Read the model definition and answer for the solid it produces. Units are mm, in the model's axes. Face numbers are marked on the shaded views. A direction names the side the tool comes from. Round coordinates to 2 decimals unless told otherwise and drop trailing zeros. Write each loop counter-clockwise with the first axis right and the second up, starting at its lowest first coordinate (ties: lowest second). Pieces come first, ordered by that corner, then holes. Notation, with made-up numbers: (52, 37) - (102, 37) arc R25 ccw to (102, 55) - close; hole circle Ø2 at (21, -32.5). An arc over 180 degrees is marked (long way). Answer as CSV lines item,"result". Start each with the question number.
1) Consider line 1 along Z through (x, y) = (-7.5, 9); line 2 along X through (y, z) = (10, -60); line 3 along X through (y, z) = (5.25, -22). Determine where each line is inside the solid, lowest interval first.
2) Find section B-B on z = -32. Determine the outline of the cut face in (x, y), then the cut area to 3 significant figures.
3) Find section D-D on z = -20. Determine the outline of the cut face in (x, y).
4) Find section A-A on y = 5.75. Determine the outline of the cut face in (x, z).
5) Each of these flat-tipped pins is pushed along its axis until it touches: pin 1 (1 mm diameter, centred on x = -8.5, z = -40.5, fed in from +Y); pin 2 (2.5 mm diameter, centred on y = 6.5, z = -33.5, fed in from +X); pin 3 (4 mm diameter, centred on x = -7.5, y = 8, fed in from -Z). Where does it stop, or does it pass through?
6) Which of the six approach directions +Z, -Z, +X, -X, +Y, -Y give full straight-line access (tool end or side, diameter ignored) to the marked faces 1, 2 and 3?
7) Find section C-C on x = -4.25. Determine the outline of the cut face in (y, z).
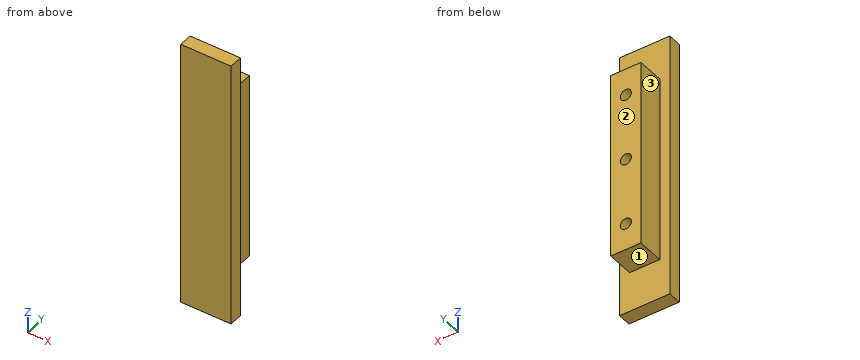
Autodesk Inventor part; units mm, degrees
ref_plane "YZ Plane" through (0, 0, 0) normal (1, 0, 0) x (0, 1, 0)
ref_plane "XZ Plane" through (0, 0, 0) normal (0, 1, 0) x (-1, 0, 0)
ref_plane "XY Plane" through (0, 0, 0) normal (0, 0, 1) x (1, 0, 0)
sketch "Sketch1" plane through (0, 0, 0) normal (0, 1, 0) x (-1, 0, 0)
  line L0 (0, 0) -> (15, 0)
  line L1 (15, 0) -> (15, -80)
  line L2 (15, -80) -> (0, -80)
  line L3 (0, -80) -> (0, 0)
  dimension "d0" = 15
  dimension "d1" = 80
extrude "Extrusion1" add sketch "Sketch1" along normal blind 4
sketch "Sketch2" plane through (0, 4, 0) normal (0, 1, 0) x (1, 0, 0)
  line L0 (-15, 80) -> (-15, 0)
  line L1 (0, 0) -> (0, 80)
  line L2 (-15, 80) -> (0, 80)
  line L3 (0, 80) -> (0, 0)
  line L4 (0, 0) -> (-15, 0)
  line L5 (-15, 0) -> (-15, 80)
  line L6 (-15, 0) -> (0, 0)
  line L7 (-15, 80) -> (-7.5, 80)
  line L8 (-7.5, 80) -> (-7.5, 0)
  line L9 (-7.5, 0) -> (-15, 0)
  line L10 (-15, 0) -> (-15, 80)
  line L11 (-7.5, 0) -> (-7.5, 20)
  line L12 (-7.5, 20) -> (-7.5, 40)
  line L13 (-7.5, 40) -> (-7.5, 60)
  circle A0 centre (-7.5, 60) radius 1.65
  circle A1 centre (-7.5, 40) radius 1.65
  circle A2 centre (-7.5, 20) radius 1.65
  line L14 (-7.5, 80) -> (-7.5, 68)
  line L15 (-7.5, 0) -> (-7.5, 12)
  line L16 (-12, 68) -> (-3, 68)
  line L17 (-3, 68) -> (-3, 12)
  line L18 (-3, 12) -> (-12, 12)
  line L19 (-12, 12) -> (-12, 68)
  dimension "d4" = 20
  dimension "d5" = 20
  dimension "d6" = 20
  dimension "d7" = 3.3
  dimension "d8" = 3.3
  dimension "d9" = 3.3
  dimension "d10" = 12
  dimension "d11" = 12
  dimension "d12" = 9
extrude "Extrusion2" add sketch "Sketch2" along normal blind 8 contours L16 L17 L18 L8 A2 A1 A0 | L8 A0 A1 A2 L18 L19 L16
sketch "Sketch3" plane through (-3, 4, -12) normal (1, 0, 0) x (0, 0, -1)
  point P0 (-12, -4)
properties part number "Pin holder"
Check values:
1,line 1,"z = -68 to -61.65, -58.35 to -41.65, -38.35 to -21.65, -18.35 to -12"
1,line 2,"x = -12 to -9.15, -5.85 to -3"
1,line 3,"x = -12 to -3"
2,outline,"(-15, 0) - (0, 0) - (0, 4) - (-3, 4) - (-3, 12) - (-12, 12) - (-12, 4) - (-15, 4) - close"
2,area,"132 mm^2"
3,outline,"(-15, 0) - (0, 0) - (0, 4) - (-3, 4) - (-3, 12) - (-5.85, 12) - (-5.85, 4) - (-9.15, 4) - (-9.15, 12) - (-12, 12) - (-12, 4) - (-15, 4) - close"
4,outline,"(-12, -68) - (-3, -68) - (-3, -12) - (-12, -12) - close; hole circle Ø3.3 at (-7.5, -60); hole circle Ø3.3 at (-7.5, -40); hole circle Ø3.3 at (-7.5, -20)"
5,pin 1,"stops at y = 4"
5,pin 2,"stops at x = -3"
5,pin 3,"stops at z = -68"
6,face 1,"-Z, +X, -X, +Y"
6,face 2,"+Z, -Z, +X, -X, +Y"
6,face 3,"+Z, -Z, -X, +Y"
7,outline,"(0, -80) - (4, -80) - (4, -68) - (12, -68) - (12, -12) - (4, -12) - (4, 0) - (0, 0) - close"
